Build history of the part. All positions in model axes, mm. Give positions to 0.01 mm unless a question says otherwise; leave off trailing zeros. Order: outer loops, then holes, each group sorted by start corner. A loop starts at its lowest first (then second) coordinate and runs counter-clockwise, first axis right, second up. Notation, with made-up numbers: (73, 7.25) -> (111, 7.25) arc R17 cw to (111, 37.25) -> close; hole circle Ø8 at (2.5, 88). An arc over 180 degrees is marked (long way). Use a Markdown table: item, result. Add a question column.
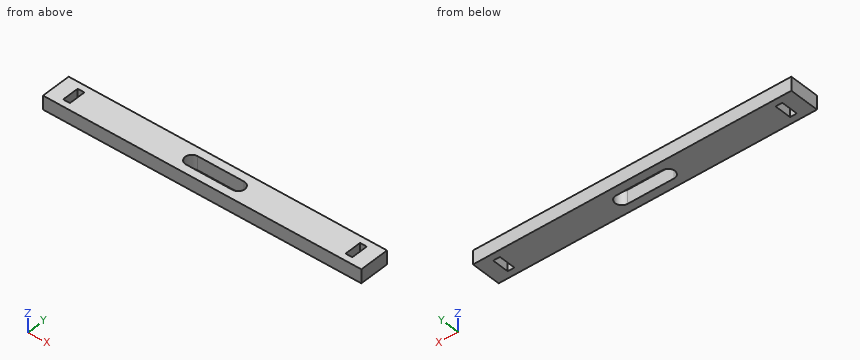
```python
from build123d import *

# Parameters (mm, degrees)
SKETCH1_W           = 72
SKETCH1_H           = 6.748944735
SKETCH1_W_2         = 1.524
SKETCH1_H_2         = 3.81
BOSS_EXTRUDE1_DEPTH = 3.1115


with BuildPart() as part:
    # Sketch1 → Boss-Extrude1 (new body)
    with BuildSketch(Plane.XY):
        with Locations((-0.032699801, 0.340407728)):
            Rectangle(SKETCH1_W, SKETCH1_H)
        with Locations((31.905300199, 0.340407728)):
            Rectangle(SKETCH1_W_2, SKETCH1_H_2, mode=Mode.SUBTRACT)
        with Locations((-31.970699801, 0.340407728)):
            Rectangle(SKETCH1_W_2, SKETCH1_H_2, mode=Mode.SUBTRACT)
        with BuildLine():
            Line((-5.27007754, 1.840407728), (5.204677939, 1.840407728))
            ThreePointArc((5.204677939, 1.840407728), (6.704677939, 0.340407728), (5.204677939, -1.159592272))
            Line((5.204677939, -1.159592272), (-5.27007754, -1.159592272))
            ThreePointArc((-5.27007754, -1.159592272), (-6.77007754, 0.340407728), (-5.27007754, 1.840407728))
        make_face(mode=Mode.SUBTRACT)
    extrude(amount=BOSS_EXTRUDE1_DEPTH)


solid = part.part
```
(1) Band-saw the part on B-B on y = 1. Give the cut face in (x, z).
(2) Band-saw the part on A-A on z = 2.45. Give the cut face in (x, y), plus the area to 3 significant figures.
(3) Wall check: probe 1 along X at (y, z) = (0.5, 1.3); probe 2 along X at (y, z) = (0, 1.6); probe 3 along Y at (x, z) = (-32.5, 0.25). Give the ranges that are in metal, low to high.
Response:
| question | item | result |
|---|---|---|
| 1 | outline | (-36.03, 0) -> (-32.73, 0) -> (-32.73, 3.11) -> (-36.03, 3.11) -> close; (-31.21, 0) -> (-6.62, 0) -> (-6.62, 3.11) -> (-31.21, 3.11) -> close; (6.55, 0) -> (31.14, 0) -> (31.14, 3.11) -> (6.55, 3.11) -> close; (32.67, 0) -> (35.97, 0) -> (35.97, 3.11) -> (32.67, 3.11) -> close |
| 2 | outline | (-36.03, -3.03) -> (35.97, -3.03) -> (35.97, 3.71) -> (-36.03, 3.71) -> close; hole (-32.73, -1.56) -> (-31.21, -1.56) -> (-31.21, 2.25) -> (-32.73, 2.25) -> close; hole (-5.27, -1.16) -> (5.2, -1.16) arc R1.5 ccw to (5.2, 1.84) -> (-5.27, 1.84) arc R1.5 ccw to start; hole (31.14, -1.56) -> (32.67, -1.56) -> (32.67, 2.25) -> (31.14, 2.25) -> close |
| 2 | area | 436 mm² |
| 3 | probe 1 | x = -36.03 to -32.73, -31.21 to -6.76, 6.7 to 31.14, 32.67 to 35.97 |
| 3 | probe 2 | x = -36.03 to -32.73, -31.21 to -6.73, 6.67 to 31.14, 32.67 to 35.97 |
| 3 | probe 3 | y = -3.03 to -1.56, 2.25 to 3.71 |
